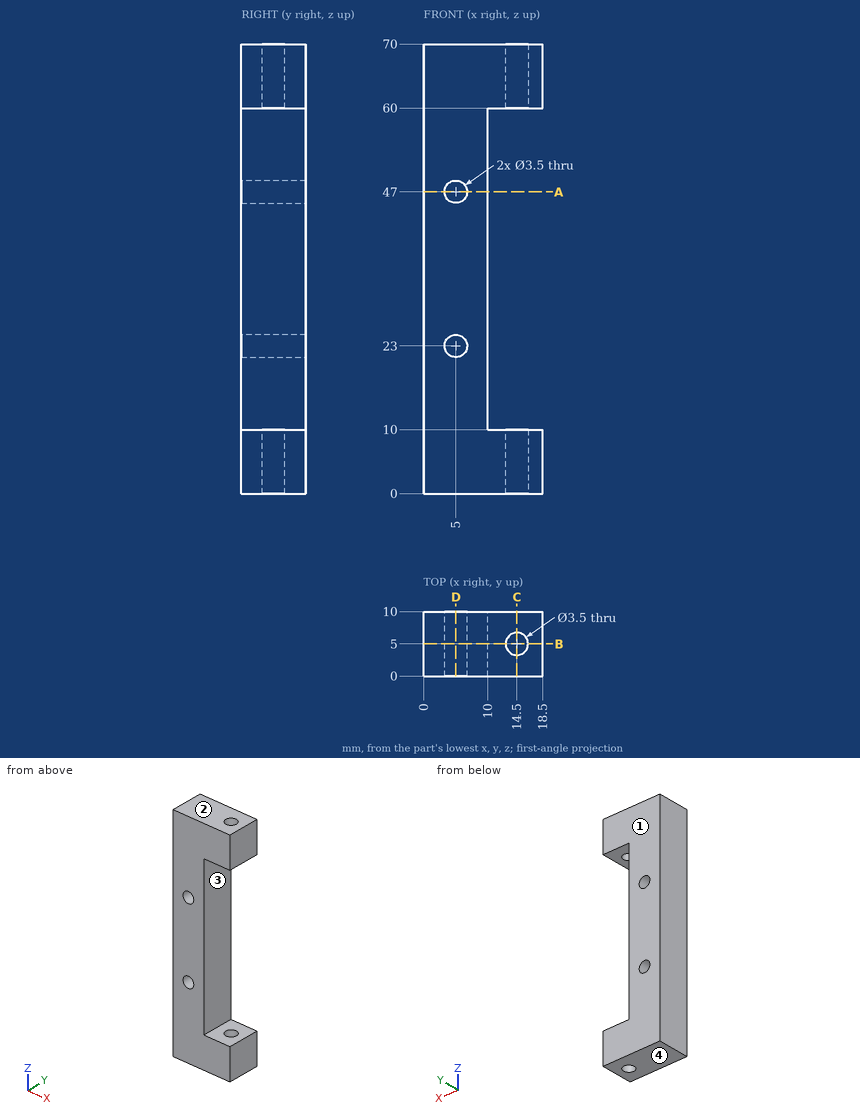
Print and shaded views of the part. All mm, measured from the part's lowest x, y and z. Give positions to 0.01 mm unless a question says otherwise; leave off trailing zeros. Loops run counter-clockwise (first coordinate to the right, second up) from the corner with the lowest first, then second, coordinate; pieces in that order, holes last. Notation, with made-up numbers: (28, 64.5) -> (34, 64.5) arc R28 ccw to (34, 95.5) -> close; hole circle Ø10 at (78, 68.5). An arc over 180 degrees is marked (long way). One line per question, with ' | ' between items. Start each with the question number.
1) Cut at B-B (y = 5). Give the cut face in (x, z), plus the area to 3 significant figures.
2) Cut at A-A (z = 47). Give the cut face in (x, y), plus the area to 3 significant figures.
3) Two-plate mould, pull along Z, no slides. Class the marked faces 1, 2, 3 and 4: released by +Z, released by -Z, zero draft, split by the parting line, or undercut.
4) Cut at D-D (x = 5). Give the cut face in (y, z), plus the area to 3 significant figures.
5) Pin check, flat tips, straight feed: pin 1 (4 mm diameter, centred on x = 14.5, y = 6, fed in from +Z); pin 2 (5 mm diameter, centred on y = 6, z = 45.5, fed in from +X). Stop position of each tip, or through.
6) Cut at C-C (x = 14.5). Give the cut face in (y, z), plus the area to 3 significant figures.
7) Probe L1, parallel to X at y = 4.25, z = 47; L2, parallel to Z at x = 10.5, y = 1.75. List the from-to ranges inside material, lowest first.
Return value:
1) outline: (0, 0) -> (12.75, 0) -> (12.75, 10) -> (10, 10) -> (10, 60) -> (12.75, 60) -> (12.75, 70) -> (0, 70) -> close; (16.25, 0) -> (18.5, 0) -> (18.5, 10) -> (16.25, 10) -> close; (16.25, 60) -> (18.5, 60) -> (18.5, 70) -> (16.25, 70) -> close; hole circle Ø3.5 at (5, 23); hole circle Ø3.5 at (5, 47) | area: 781 mm^2
2) outline: (0, 0) -> (3.25, 0) -> (3.25, 10) -> (0, 10) -> close; (6.75, 0) -> (10, 0) -> (10, 10) -> (6.75, 10) -> close | area: 65.0 mm^2
3) face 1: zero draft | face 2: released by +Z | face 3: undercut | face 4: released by -Z
4) outline: (0, 0) -> (10, 0) -> (10, 21.25) -> (0, 21.25) -> close; (0, 24.75) -> (10, 24.75) -> (10, 45.25) -> (0, 45.25) -> close; (0, 48.75) -> (10, 48.75) -> (10, 70) -> (0, 70) -> close | area: 630 mm^2
5) pin 1: z = 70 | pin 2: x = 10
6) outline: (0, 0) -> (3.25, 0) -> (3.25, 10) -> (0, 10) -> close; (0, 60) -> (3.25, 60) -> (3.25, 70) -> (0, 70) -> close; (6.75, 0) -> (10, 0) -> (10, 10) -> (6.75, 10) -> close; (6.75, 60) -> (10, 60) -> (10, 70) -> (6.75, 70) -> close | area: 130 mm^2
7) L1: 0 to 3.25, 6.75 to 10 | L2: 0 to 10, 60 to 70
